Source: CAD feature listing. Evaluate the final solid. Frame: model axes, mm. Face numbers are marked on the shaded views. Give positions to 0.01 mm unless a question says otherwise; leave off trailing zeros. Order: outer loops, then holes, each group sorted by start corner. A loop starts at its lowest first (then second) coordinate and runs counter-clockwise, first axis right, second up. Notation, with made-up numbers: (20, 82) -> (77, 82) arc R29 cw to (77, 107) -> close; hole circle Ø6 at (30.25, 54.25). An arc over 180 degrees is marked (long way). Use CSV: the item, a comma, the result in double quotes.
```python
from build123d import *

# Parameters (mm, degrees)
CROQUIS1_R                        = 44
CROQUIS1_R_2                      = 40
MANGA_DEPTH                       = 13
CROQUIS2_R                        = 44
CROQUIS2_R_2                      = 36
LABIO_DEPTH                       = 10
PASANTES_M3_RADIALES_A_DEPTH      = 67.340033162
PASANTES_M3_RADIALES_A_DEPTH_BACK = 67.340033162
CROQUIS3_R                        = 1.7
PASANTES_M3_RADIALES_B_DEPTH      = 67.340033339
PASANTES_M3_RADIALES_B_DEPTH_BACK = 67.340033339
CROQUIS4_R                        = 1.7
CROQUIS10_W                       = 3.5
CROQUIS10_H                       = 6.8
CROQUIS10_W_2                     = 6.8
CROQUIS10_H_2                     = 3.5
PLANOS_M3_TORNILLOS_DEPTH         = 6.8


with BuildPart() as part:
    # Croquis1 → Manga (new body)
    with BuildSketch(Plane.XY):
        with Locations(Location((0, 0, 0), (0, 0, 180))):
            Circle(CROQUIS1_R)
        with Locations(Location((0, 0, 0), (0, 0, 180))):
            Circle(CROQUIS1_R_2, mode=Mode.SUBTRACT)
    extrude(amount=MANGA_DEPTH)

    # Croquis2 → Labio (add)
    with BuildSketch(Plane.XY.offset(13)):
        with Locations(Location((0, 0, 0), (0, 0, 180))):
            Circle(CROQUIS2_R)
        Circle(CROQUIS2_R_2, mode=Mode.SUBTRACT)
    extrude(amount=LABIO_DEPTH)

    # Croquis3 → Pasantes_M3_radiales_A (cut, two sides: drawn at the far end of the back side and taken through both)
    with BuildSketch(Plane(origin=(0, 0, 0), x_dir=(1, 0, 0), z_dir=(0, 1, 0)).offset(-PASANTES_M3_RADIALES_A_DEPTH_BACK)):
        with Locations(Location((0, -7, 0), (0, 0, 270))):
            Circle(CROQUIS3_R)
    extrude(amount=PASANTES_M3_RADIALES_A_DEPTH + PASANTES_M3_RADIALES_A_DEPTH_BACK, mode=Mode.SUBTRACT)

    # Croquis4 → Pasantes_M3_radiales_B (cut, two sides: drawn at the far end of the back side and taken through both)
    with BuildSketch(Plane(origin=(0, 0, 0), x_dir=(0, 0, -1), z_dir=(1, 0, 0)).offset(-PASANTES_M3_RADIALES_B_DEPTH_BACK)):
        with Locations((-7, 0)):
            Circle(CROQUIS4_R)
    extrude(amount=PASANTES_M3_RADIALES_B_DEPTH + PASANTES_M3_RADIALES_B_DEPTH_BACK, mode=Mode.SUBTRACT)

    # Croquis10 → Planos_M3_tornillos (cut)
    with BuildSketch(Plane.XY.offset(3.6)):
        with Locations((43.75, 0)):
            Rectangle(CROQUIS10_W, CROQUIS10_H)
        with Locations((0, 43.75)):
            Rectangle(CROQUIS10_W_2, CROQUIS10_H_2)
        with Locations((-43.75, 0)):
            Rectangle(CROQUIS10_W, CROQUIS10_H)
        with Locations((0, -43.75)):
            Rectangle(CROQUIS10_W_2, CROQUIS10_H_2)
    extrude(amount=PLANOS_M3_TORNILLOS_DEPTH, mode=Mode.SUBTRACT)


solid = part.part
```
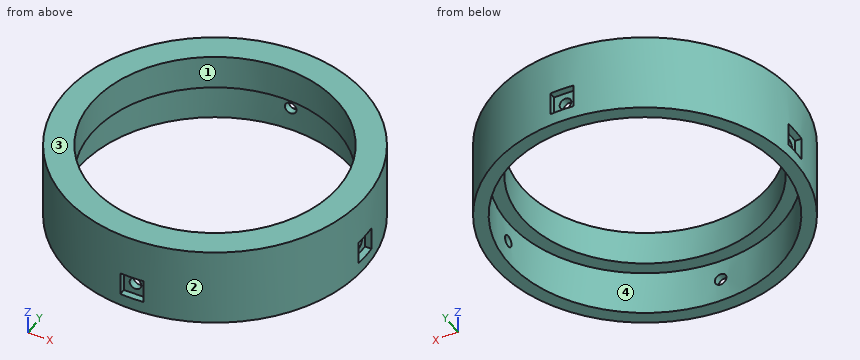
1. Section query B-B on x = 0. Return loops of the section in (y, z), plus the area to 3 significant figures.
Answer below:
outline,"(-44, 0) -> (-40, 0) -> (-40, 5.3) -> (-42, 5.3) -> (-42, 3.6) -> (-44, 3.6) -> close; (-44, 10.4) -> (-42, 10.4) -> (-42, 8.7) -> (-40, 8.7) -> (-40, 13) -> (-36, 13) -> (-36, 23) -> (-44, 23) -> close; (36, 13) -> (40, 13) -> (40, 8.7) -> (42, 8.7) -> (42, 10.4) -> (44, 10.4) -> (44, 23) -> (36, 23) -> close; (40, 0) -> (44, 0) -> (44, 3.6) -> (42, 3.6) -> (42, 5.3) -> (40, 5.3) -> close"
area,"223 mm²"
2. Mould query, pull axis X, two halves, no side actions, for the marked faces 1, 2, 3 and 4. Classes: released by +X, released by -X, zero draft, split by the parting line, or undercut.
Answer below:
face 1,"undercut"
face 2,"split by the parting line"
face 3,"zero draft"
face 4,"undercut"
3. Pin query (flat end, axial travel): P1, Ø10, axis at y = 33.5, z = 20.5, coming from the +X side; P2, Ø4, axis at y = -15, z = 8.5, coming from the -X side; P3, Ø8, axis at x = 14, z = 20.5, coming from the +Y side. Return the tip coordinate at first contact, or that it passes through.
Answer below:
P1,"stops at x = 33.52"
P2,"stops at x = -42.04"
P3,"stops at y = 42.85"
4. Section query D-D on x = 27.5. Return loops of the section in (y, z), plus the area to 3 significant figures.
Answer below:
outline,"(-34.35, 0) -> (-29.05, 0) -> (-29.05, 13) -> (-23.23, 13) -> (-23.23, 23) -> (-34.35, 23) -> close; (23.23, 13) -> (29.05, 13) -> (29.05, 0) -> (34.35, 0) -> (34.35, 23) -> (23.23, 23) -> close"
area,"360 mm²"
5. Ray query, line 1 along Z through (x, y) = (0, 41); line 2 along Y through (x, z) = (0, 17); line 3 along Z through (x, y) = (16, -35.5). Return the intervals inside material, ascending.
Answer below:
line 1,"z = 0 to 5.3, 8.7 to 23"
line 2,"y = -44 to -36, 36 to 44"
line 3,"z = 13 to 23"
6. Section query A-A on z = 7. Count the separate pieces of the cut face and the enclosed holes in it, plus the area to 3 significant figures.
Answer below:
separate pieces,"4"
enclosed holes,"0"
area,"975 mm²"
